from build123d import *

# Parameters (mm, degrees)
BOSS_EXTRUDE1_DEPTH  = 1.6
M3_CLEARANCE_HOLE1_D = 3.4


with BuildPart() as part:
    # Sketch5 → Boss-Extrude1 (new body)
    with BuildSketch(Plane(origin=(9.507139376, -10.778899957, 0), x_dir=(0, 0, -1), z_dir=(0.661478652, -0.749963994, 0))):
        Polygon((-18.324577301, 51.705324763), (21.675422699, 51.705324763), (18.090793802, 40.16602452), (16.562821188, 40.640681966), (12.673658844, 28.121056286), (14.201631457, 27.64639884), (10.675422699, 16.295159211), (9, 16.295159211), (-7.324577301, 16.295159211), (-10.991243968, 28.098547728), (-12.519216582, 27.623890282), (-16.185883249, 39.427278799), (-14.657910635, 39.901936245), align=None)
    extrude(amount=BOSS_EXTRUDE1_DEPTH)

    # M3 Clearance Hole1 (through all)
    with Locations(Plane(origin=(9.507139376, -10.778899957, 0), x_dir=(0.749963994, 0.661478652, 0), z_dir=(-0.661478652, 0.749963994, 0))):
        with Locations((19.295159211, 0.837711349)):
            Hole(M3_CLEARANCE_HOLE1_D / 2)


solid = part.part
Input: part model. Units: mm. Frame: model coordinates. A direction names the side the tool comes from. Coordinates: 2 decimals unless noted, no trailing zeros. Loops run counter-clockwise (first coordinate to the right, second up) from the corner with the lowest first, then second, coordinate; pieces in that order, holes last.
Q1. Set-up query: faces 1 (the face through (39.773, 14.865, 15.433)), 2 (the face through (39.201, 13.278, -1.955)). Return all of +Z, -Z, +X, -X, +Y, -Y with unobstructed straight access to the full face (end or side cutting, diameter ignored); none if empty.
Q2. Material intervals for line 1 (X direction, y = 19.75, z = -18); line 2 (Z direction, x = 27.5, y = 4.75); line 3 (X direction, y = 4, z = 9), sorted ascending.
Q3. Cut plane B-B (y = 10). Output: boundary loops of the cut face in (x, z), then the cut area to 3 significant figures.
Q4. Draft query along Z for faces 3 (the face through (44.318, 18.873, 16.466)), 4 (the face through (40.3, 15.4, -17.3)), 5 (the face through (30.93, 7.06, 11.74)), 6 (the face through (30.94, 7.08, -13.43)). Return one class per face: +Z half, -Z half, draft (parallel to the pull), parting line (faces both ways), or undercut.
Q5. Contact query for flat-ended pins moving along their axis: pin 1 (5 mm diameter, centred on x = 34.5, z = 4, fed in from -Y); pin 2 (8 mm diameter, centred on x = 40.5, z = 1, fed in from -Y); pin 3 (2 mm diameter, centred on y = 6.5, z = 1, fed in from -X). Output: stop coordinate, or through.
Q6. Cut plane A-A (z = -9). Output: boundary loops of the cut face in (x, y).
Working result:
1. face 1: +Z
1. face 2: +Z, -Z, +X, -Y
2. line 1: x = 44.12 to 46.54
2. line 2: z = -13 to 9.65
2. line 3: x = 26.26 to 28.68
3. outline: (33.07, -13.7) - (35.48, -14.26) - (35.48, 14.26) - (33.07, 13.7) - close
3. area: 67.6 mm2
4. face 3: +Z half
4. face 4: undercut
4. face 5: undercut
4. face 6: -Z half
5. pin 1: stops at y = 6.93
5. pin 2: stops at y = 10.9
5. pin 3: stops at x = 27.96
6. outline: (21.73, 0) - (22.79, -1.2) - (49.34, 22.22) - (48.28, 23.42) - close
